```python
from build123d import *

# Parameters (mm, degrees)
SKETCH_1_W          = 29
SKETCH_1_H          = 57
SKETCH_1_R          = 1.45
SKETCH_1_W_2        = 21
SKETCH_1_H_2        = 41
EXTRUDE_1_DEPTH     = 28
SKETCH_2_W          = 25
SKETCH_2_H          = 26
CUT_EXTRUDE_1_DEPTH = 7
SKETCH_3_W          = 49
SKETCH_3_H          = 26
CUT_EXTRUDE_2_DEPTH = 25
SKETCH_4_W          = 4
SKETCH_4_H          = 41
CUT_EXTRUDE_3_DEPTH = 25
FILLET_1_R          = 2
SKETCH_5_W          = 50
SKETCH_5_H          = 90
EXTRUDE_2_DEPTH     = 3


with BuildPart() as part:
    # 스케치1 → 보스-돌출1 (new body)
    with BuildSketch(Plane(origin=(0, 0, 0), x_dir=(1, 0, 0), z_dir=(0, 1, 0))):
        Rectangle(SKETCH_1_W, SKETCH_1_H)
        with Locations(Location((-5, 24.31, 0), (0, 0, 270))):
            Circle(SKETCH_1_R, mode=Mode.SUBTRACT)
        with Locations(Location((-5, -24.32, 0), (0, 0, 270))):
            Circle(SKETCH_1_R, mode=Mode.SUBTRACT)
        with Locations(Location((5, -24.32, 0), (0, 0, 90))):
            Circle(SKETCH_1_R, mode=Mode.SUBTRACT)
        with Locations(Location((5, 24.31, 0), (0, 0, 90))):
            Circle(SKETCH_1_R, mode=Mode.SUBTRACT)
        Rectangle(SKETCH_1_W_2, SKETCH_1_H_2, mode=Mode.SUBTRACT)
    extrude(amount=EXTRUDE_1_DEPTH)

    # 스케치2 → 컷-돌출1 (cut)
    with BuildSketch(Plane(origin=(-14, 0, 28.5), x_dir=(-1, 0, 0), z_dir=(0, 0, -1))):
        with Locations((-14, 13)):
            Rectangle(SKETCH_2_W, SKETCH_2_H)
    extrude(amount=CUT_EXTRUDE_1_DEPTH, mode=Mode.SUBTRACT)

    # 스케치3 → 컷-돌출2 (cut)
    with BuildSketch(Plane(origin=(14.5, 0, 0), x_dir=(0, 0, -1), z_dir=(1, 0, 0))):
        with Locations((4, 13)):
            Rectangle(SKETCH_3_W, SKETCH_3_H)
    extrude(amount=-CUT_EXTRUDE_2_DEPTH, mode=Mode.SUBTRACT)

    # 스케치4 → 컷-돌출3 (cut)
    with BuildSketch(Plane(origin=(0, 28, 0), x_dir=(1, 0, 0), z_dir=(0, 1, 0))):
        with Locations((12.5, 0)):
            Rectangle(SKETCH_4_W, SKETCH_4_H)
    extrude(amount=-CUT_EXTRUDE_3_DEPTH, mode=Mode.SUBTRACT)

    # 필렛1
    fillet_1_edges = [part.edges().sort_by_distance(p)[0] for p in [
        (-10.5, 26, -24.5),
    ]]
    fillet(fillet_1_edges, radius=FILLET_1_R)

    # 스케치5 → 보스-돌출2 (add)
    with BuildSketch(Plane.XZ):
        with Locations((0, -10.4)):
            Rectangle(SKETCH_5_W, SKETCH_5_H)
    extrude(amount=EXTRUDE_2_DEPTH)


solid = part.part
```
For this review, take the finished solid that the model builds, in its own axes (mm). A direction names the side the tool comes from. Round coordinates to 2 decimals unless told otherwise and drop trailing zeros. Write each loop counter-clockwise with the first axis right and the second up, starting at its lowest first coordinate (ties: lowest second). Pieces come first, ordered by that corner, then holes. Notation, with made-up numbers: (8.5, 84) - (57.5, 84) arc R17 cw to (57.5, 99) - close; hole circle Ø2 at (-28.5, 58.5). An arc over 180 degrees is marked (long way). Use CSV: the item, a comma, the result in double quotes.
1) For faces 5 (the flat face through (0, 26, 25)), 6 (the flat face through (-14.5, 14, 0)), 7 (the cylindrical face through (-4.94, 26.99, -25.76)), list the 3-axis set-ups (+Z, -Z, +X, -X, +Y, -Y) from which the entire face can be reached by the end or side of a thin tool; tool diameter is ignored.
Conclusion:
face 5,"+Z"
face 6,"+Z, -Z, -X, +Y"
face 7,"+Y"
2) Wall thickness on line 1 along Z through (x, y) = (-5, 27.4); line 2 along X through (y, z) = (26.9, 24.32); line 3 along Y through (x, z) = (-3, 18): over which ranges is each line inside the solid? List them lowest first. Write a range as from..to.
Conclusion:
line 1,"z = -28.5..-25.76, -22.86..-20.5, 20.5..22.87, 25.77..28.5"
line 2,"x = -14.5..-6.45, -3.55..3.55, 6.45..14.5"
line 3,"y = -3..0"
3) Add section B-B on x = -5. Write out the cut boundary in (y, z), and give its area (3 significant figures).
Conclusion:
outline,"(-3, -55.4) - (0, -55.4) - (0, 20.5) - (28, 20.5) - (28, 22.87) - (26, 22.87) - (26, 21.5) - (0, 21.5) - (0, 34.6) - (-3, 34.6) - close; (26, -28.5) - (28, -28.5) - (28, -25.76) - (26, -25.76) - close; (26, -22.86) - (28, -22.86) - (28, -20.5) - (26, -20.5) - close; (26, 25.77) - (28, 25.77) - (28, 28.5) - (26, 28.5) - close"
area,"316 mm^2"
4) Add section A-A on z = -24.31. Write out the cut boundary in (x, y).
Conclusion:
outline,"(-25, -3) - (25, -3) - (25, 0) - (-10.5, 0) - (-10.5, 24) arc R2 cw to (-8.5, 26) - (-6.45, 26) - (-6.45, 28) - (-14.5, 28) - (-14.5, 0) - (-25, 0) - close; (-3.55, 26) - (3.55, 26) - (3.55, 28) - (-3.55, 28) - close; (6.45, 26) - (14.5, 26) - (14.5, 28) - (6.45, 28) - close"
5) Add section D-D on y = 12. Write out the cut boundary in (x, z), and give its area (3 significant figures).
Conclusion:
outline,"(-14.5, -28.5) - (-10.5, -28.5) - (-10.5, 20.5) - (14.5, 20.5) - (14.5, 28.5) - (12.5, 28.5) - (12.5, 21.5) - (-12.5, 21.5) - (-12.5, 28.5) - (-14.5, 28.5) - close"
area,"253 mm^2"
6) The part is to be moulded in two halves that separate along X. For faces 1 (the flat face through (-25, -1, -11)), 2 (the cylindrical face through (4.02, 26.99, -23.24)), 3 (the cylindrical face through (-9.9, 25.43, -24.56)), 4 (the flat face through (0, -1, -55.4)), say which applies: pulls with the +X half, pulls with the -X half, needs draft (parallel to the pull), parting line crosses it, or undercut.
Conclusion:
face 1,"pulls with the -X half"
face 2,"undercut"
face 3,"pulls with the +X half"
face 4,"needs draft"
7) Add section C-C on z = 24.32. Write out the cut boundary in (x, y), and give its area (3 significant figures).
Conclusion:
outline,"(-25, -3) - (25, -3) - (25, 0) - (14.5, 0) - (14.5, 28) - (6.45, 28) - (6.45, 26) - (12.5, 26) - (12.5, 0) - (-12.5, 0) - (-12.5, 26) - (-6.45, 26) - (-6.45, 28) - (-14.5, 28) - (-14.5, 0) - (-25, 0) - close; (-3.55, 26) - (3.55, 26) - (3.55, 28) - (-3.55, 28) - close"
area,"300 mm^2"
8) Clearance check with flat-ended pins moving along their axes: pin 1 Ø10 at (y, z) = (18.5, -26.5) entering from -X; pin 2 Ø3 at (x, y) = (5, 25.5) entering from +Z; pin 3 Ø4 at (y, z) = (16.5, 23) entering from +X; pin 4 Ø1 at (y, z) = (1.5, -42) entering from -X. State where each tip first meets the part, or that it passes through.
Conclusion:
pin 1,"stops at x = -14.5"
pin 2,"stops at z = 28.5"
pin 3,"stops at x = 14.5"
pin 4,"passes through"
